Study the drawing (mm; zero at the part's minimum x, y, z) and answer. Coordinates: 2 decimals unless noted, no trailing zeros. Write each loop counter-clockwise with the first axis right and the second up, starting at its lowest first coordinate (ties: lowest second). Pieces come first, ordered by that corner, then holes. Notation, with made-up numbers: (38.5, 41) - (58.5, 41) arc R28 ccw to (58.5, 59) - close; hole circle Ø4 at (9.25, 34). An arc over 180 degrees is marked (long way). One line per item, written item: value.
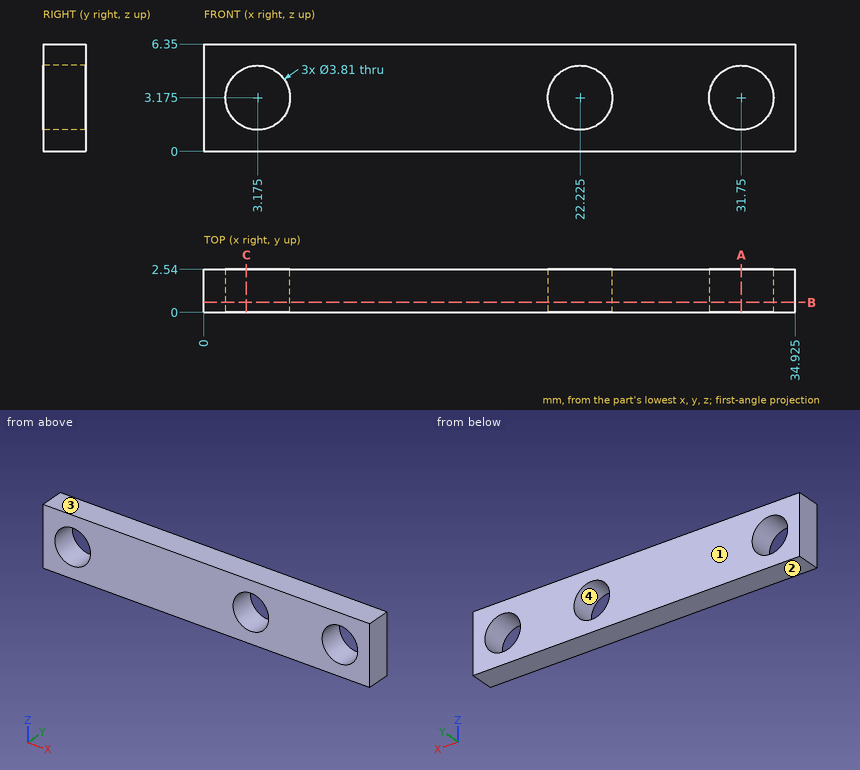
Item 1: Consider probe 1 along Z at (x, y) = (31.75, 1.15); probe 2 along X at (y, z) = (2.3, 3.5) (3 decimals); probe 3 along X at (y, z) = (1.3, 2.75) (3 decimals). Determine where each line is inside the solid, lowest interval first.
Evaluation:
probe 1: z = 0 to 1.27, 5.08 to 6.35
probe 2: x = 0 to 1.298, 5.052 to 20.348, 24.102 to 29.873, 33.627 to 34.925
probe 3: x = 0 to 1.318, 5.032 to 20.368, 24.082 to 29.893, 33.607 to 34.925
Item 2: Section A-A, the plane x = 31.75 is taken. Determine the outline of the cut face in (y, z), then the cut area to 3 significant figures.
Evaluation:
outline: (0, 0) - (2.54, 0) - (2.54, 1.27) - (0, 1.27) - close; (0, 5.08) - (2.54, 5.08) - (2.54, 6.35) - (0, 6.35) - close
area: 6.45 mm2
Item 3: Section B-B, the plane y = 0.6 is taken. Determine the outline of the cut face in (x, z) (3 decimals), then the cut area to 3 significant figures.
Evaluation:
outline: (0, 0) - (34.925, 0) - (34.925, 6.35) - (0, 6.35) - close; hole circle Ø3.81 at (3.175, 3.175); hole circle Ø3.81 at (22.225, 3.175); hole circle Ø3.81 at (31.75, 3.175)
area: 188 mm2
Item 4: Section C-C, the plane x = 2.5 is taken. Determine the outline of the cut face in (y, z).
Evaluation:
outline: (0, 0) - (2.54, 0) - (2.54, 1.39) - (0, 1.39) - close; (0, 4.96) - (2.54, 4.96) - (2.54, 6.35) - (0, 6.35) - close
Item 5: Determine the mould class of the marked faces 1, 2, 3 and 4 for opening direction Z: +Z half, -Z half, draft (parallel to the pull), parting line (faces both ways), or undercut.
Evaluation:
face 1: draft
face 2: -Z half
face 3: +Z half
face 4: undercut
